CAD build for the part. Positions are in the model's coordinates, mm. Face numbers are marked on the shaded views. Coordinates: 2 decimals unless noted, no trailing zeros. Order: outer loops, then holes, each group sorted by start corner. A loop starts at its lowest first (then second) coordinate and runs counter-clockwise, first axis right, second up. Notation, with made-up numbers: M 70,26 L 123,26 A6 ccw 123,31 Z; hole C 0,-5.5 d9. An arc over 180 degrees is marked long. Write item = value, one per line.
from build123d import *

# Parameters (mm, degrees)
SKETCH1_R               = 73.025
SKETCH1_R_2             = 69.85
BOSS_EXTRUDE1_DEPTH     = 63.5
SKETCH2_R               = 73.025
BOSS_EXTRUDE2_DEPTH     = 6.35
BOSS_EXTRUDE3_DEPTH     = 63.5
CUT_EXTRUDE2_START      = -6.35
CUT_EXTRUDE2_DEPTH      = 6.35
CUT_EXTRUDE2_DEPTH_BACK = 57.15
CUT_EXTRUDE5_DEPTH      = 1016


with BuildPart() as part:
    # Sketch1 → Boss-Extrude1 (new body)
    with BuildSketch(Plane(origin=(0, 0, 0), x_dir=(1, 0, 0), z_dir=(0, 1, 0))):
        Circle(SKETCH1_R)
        Circle(SKETCH1_R_2, mode=Mode.SUBTRACT)
    extrude(amount=BOSS_EXTRUDE1_DEPTH)

    # Sketch2 → Boss-Extrude2 (add)
    with BuildSketch(Plane.XZ):
        Circle(SKETCH2_R)
    extrude(amount=BOSS_EXTRUDE2_DEPTH)

    # Sketch3 → Boss-Extrude3 (add)
    with BuildSketch(Plane(origin=(0, 0, 0), x_dir=(1, 0, 0), z_dir=(0, 1, 0))):
        with BuildLine():
            Line((-67.615293174, -17.526968618), (-21.409243237, 66.488095205))
            ThreePointArc((-21.409243237, 66.488095205), (-61.204368783, 33.660774529), (-67.615293174, -17.526968618))
        make_face()
    extrude(amount=BOSS_EXTRUDE3_DEPTH)

    # Sketch4 → Cut-Extrude2 (cut, two sides)
    with BuildSketch(Plane(origin=(0, 63.5, 0), x_dir=(1, 0, 0), z_dir=(0, 1, 0)).offset(CUT_EXTRUDE2_START)) as cut_extrude2_sk:
        with BuildLine():
            Line((-25.79189716, 64.913793148), (-68.632882923, -12.982676212))
            ThreePointArc((-68.632882923, -12.982676212), (-61.204368783, 33.660774529), (-25.79189716, 64.913793148))
        make_face()
    extrude(amount=CUT_EXTRUDE2_DEPTH, mode=Mode.SUBTRACT)
    extrude(cut_extrude2_sk.sketch, amount=-CUT_EXTRUDE2_DEPTH_BACK, mode=Mode.SUBTRACT)

    # Sketch7 → Cut-Extrude5 (cut)
    with BuildSketch(Plane(origin=(0, 63.5, 0), x_dir=(1, 0, 0), z_dir=(0, 1, 0))):
        Polygon((-72.609628953, -26.608018388), (-10.171407592, 86.921512047), (114.959945388, 65.80584256), (122.548753565, -33.748740716), (41.017949176, -93.980716613), (-75.603403444, -72.676842996), align=None)
    extrude(amount=-CUT_EXTRUDE5_DEPTH, mode=Mode.SUBTRACT)


solid = part.part
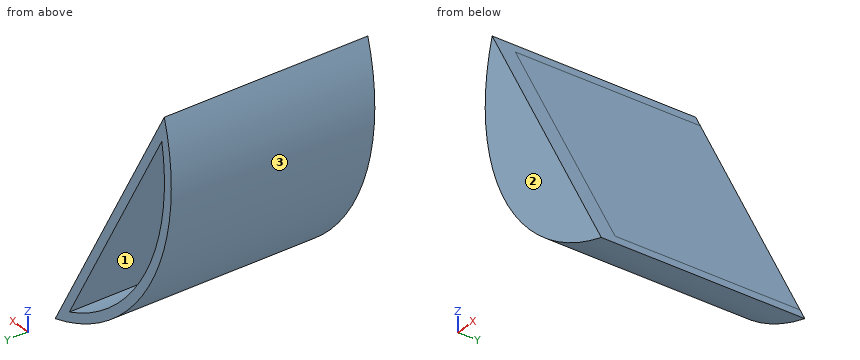
(1) Slice it at B-B, the plane z = -22. Write the cut outline in (x, y).
Evaluation:
outline = M -69.63,-6.35 L -45.88,-6.35 L -45.88,63.5 L -49.39,63.5 L -49.39,0 L -66.29,0 L -66.29,63.5 L -69.63,63.5 Z
(2) Pin check, flat tips, straight feed: pin 1 Ø5 at (x, y) = (-63, 45) entering from -Z (3 decimals); pin 2 Ø3 at (x, z) = (-62, -26.5) entering from +Y; pin 3 Ø4 at (y, z) = (31, -4) entering from +X; pin 4 Ø6 at (x, z) = (-61, 9.5) entering from +Y. Stop position of each tip, or through.
Evaluation:
pin_1 = -40.895
pin_2 = 0
pin_3 = -54.68
pin_4 = 63.5
(3) Slice it at C-C, the plane x = -36. Write the cut outline in (y, z), then the cut area to 3 significant figures.
Evaluation:
outline = M -6.35,-63.53 L 63.5,-63.53 L 63.5,-59.86 L 0,-59.86 L 0,-46.35 L 63.5,-46.35 L 63.5,-39.96 L -6.35,-39.96 Z
area = 789 mm²
(4) Slice it at A-A, the plane y = 13. Write the cut outline in (x, z) (3 decimals).
Evaluation:
outline = M -69.793,21.486 A73.025 ccw -19.232,-70.447 Z; hole M -68.633,12.983 A69.85 ccw -25.792,-64.914 Z
(5) Pull direction X, two halves, no side cores. Call the marked faces 1, 2 and 3: +X half, -X half, draft (parallel to the pull), parting line (faces both ways), or undercut.
Evaluation:
face_1 = undercut
face_2 = draft
face_3 = -X half
(6) Wall check: line 1 (X direction, y = 15.5, z = -37); line 2 (X direction, y = 58.5, z = -27.5); line 3 (Z direction, x = -51, y = 45). Give the ranges that are in metal, low to high. Write a range as from..to.
Evaluation:
line_1 = -62.96..-59.25, -41.14..-37.63
line_2 = -67.65..-64.21, -46.37..-42.85
line_3 = -52.27..-47.73, -19.08..-12.68
(7) Slice it at D-D, the plane x = -24. Write the cut outline in (y, z).
Evaluation:
outline = M -6.35,-68.97 L 63.5,-68.97 L 63.5,-61.78 L -6.35,-61.78 Z
